Work out the finished part from the listing and answer in its coordinate system (mm). A direction names the side the tool comes from. Round coordinates to 2 decimals unless told otherwise and drop trailing zeros. Loops run counter-clockwise (first coordinate to the right, second up) from the corner with the lowest first, then second, coordinate; pieces in that order, holes last.
```python
from build123d import *

# Parameters (mm, degrees)
SKETCH_2_R          = 10
CUT_EXTRUDE_2_DEPTH = 13.84610836
CHAMFER_1_SIZE      = 0.3


with BuildPart() as part:
    # Эскиз1 → Повернуть1 (revolve)
    with BuildSketch(Plane(origin=(0, 0, 0), x_dir=(1, 0, 0), z_dir=(0, 1, 0)), mode=Mode.PRIVATE) as revolve_1_sk:
        Polygon((4.3, -7.45), (6.4, -7.45), (7.4, -6.45), (7.4, 0), (5.65, 0), (5.65, -5.75), (5.35, -5.75), (5.35, -6.8), (4.3, -6.8), align=None)
    revolve(revolve_1_sk.sketch.rotate(Axis((0, 0, 0), (0, 0, 1)), 180), axis=Axis((0, 0, 0), (0, 0, 1)))

    # Эскиз2 → Вырез-Вытянуть2 (cut, through all)
    with BuildSketch(Plane.XY):
        Circle(SKETCH_2_R)
        Polygon((8.082903769, 0), (4.041451884, 7), (-4.041451884, 7), (-8.082903769, 0), (-4.041451884, -7), (4.041451884, -7), align=None, mode=Mode.SUBTRACT)
    extrude(amount=CUT_EXTRUDE_2_DEPTH, mode=Mode.SUBTRACT)

    # Фаска1
    chamfer_1_edges = [part.edges().sort_by_distance(p)[0] for p in [
        (5.65, 0, 0),
    ]]
    chamfer(chamfer_1_edges, length=CHAMFER_1_SIZE)


solid = part.part
```
1. Determine the mould class of faces 3 (the face through (1.16, 5.223, 6.282)), 4 (the face through (-3.717, -6.399, 3.18)), 5 (the face through (3.717, 6.399, 3.18)) for opening direction Y: +Y half, -Y half, draft (parallel to the pull), parting line (faces both ways), or undercut.
Answer key:
face 3: undercut
face 4: -Y half
face 5: +Y half
2. Find section D-D (z = 6). Write down the section's boundary in (x, y).
Answer key:
outline: (-7.26, -1.42) - (-4.86, -5.58) arc R7.4 ccw to (-2.4, -7) - (2.4, -7) arc R7.4 ccw to (4.86, -5.58) - (7.26, -1.42) arc R7.4 ccw to (7.26, 1.42) - (4.86, 5.58) arc R7.4 ccw to (2.4, 7) - (-2.4, 7) arc R7.4 ccw to (-4.86, 5.58) - (-7.26, 1.42) arc R7.4 ccw to start; hole circle Ø10.7 at (0, 0)
3. Find section C-C (z = 2.75). Write down the section's boundary in (x, y), then the cut area to 3 significant figures.
Answer key:
outline: (-7.26, -1.42) - (-4.86, -5.58) arc R7.4 ccw to (-2.4, -7) - (2.4, -7) arc R7.4 ccw to (4.86, -5.58) - (7.26, -1.42) arc R7.4 ccw to (7.26, 1.42) - (4.86, 5.58) arc R7.4 ccw to (2.4, 7) - (-2.4, 7) arc R7.4 ccw to (-4.86, 5.58) - (-7.26, 1.42) arc R7.4 ccw to start; hole circle Ø11.3 at (0, 0)
area: 64.0 mm2
4. Given pin 1 (1.5 mm diameter, centred on y = 1.5, z = 6, fed in from +X); pin 2 (1.5 mm diameter, centred on x = 1.5, y = 1, fed in from -Z); pin 3 (1.5 mm diameter, centred on x = -5.5, y = -4, fed in from -Z); pin 4 (3 mm diameter, centred on y = 3.5, z = 6.5, fed in from +X), each flat-ended and moving along its own axis, determine where each tip first touches the part or whether it passes through.
Answer key:
pin 1: stops at x = 7.36
pin 2: passes through
pin 3: stops at z = 0
pin 4: stops at x = 6.93
5. Consider probe 1 along Y at (x, z) = (0, 6.5); probe 2 along Y at (x, z) = (-0.75, 3.75); probe 3 along Z at (x, y) = (-6.25, -3). Determine where each line is inside the solid, lowest interval first.
Answer key:
probe 1: y = -7 to -5.35, 5.35 to 7
probe 2: y = -7 to -5.6, 5.6 to 7
probe 3: z = 0 to 6.92
6. Which of the six approach directions +Z, -Z, +X, -X, +Y, -Y give full straight-line access (tool end or side, diameter ignored) to faces 1 (the face through (-5.39, -1.7, 3.06)), 2 (the face through (0, 7, 3))?
Answer key:
face 1: -Z
face 2: +Z, -Z, +X, -X, +Y
7. Find section B-B (y = 0). Write down the section's boundary in (x, z), then the cut area to 3 significant figures.
Answer key:
outline: (-7.4, 0) - (-5.95, 0) - (-5.65, 0.3) - (-5.65, 5.75) - (-5.35, 5.75) - (-5.35, 6.8) - (-4.3, 6.8) - (-4.3, 7.45) - (-6.4, 7.45) - (-7.4, 6.45) - close; (4.3, 6.8) - (5.35, 6.8) - (5.35, 5.75) - (5.65, 5.75) - (5.65, 0.3) - (5.95, 0) - (7.4, 0) - (7.4, 6.45) - (6.4, 7.45) - (4.3, 7.45) - close
area: 27.4 mm2
8. Find section A-A (x = 0). Write down the section's boundary in (y, z), then the cut area to 4 significant figures.
Answer key:
outline: (-7, 0) - (-5.95, 0) - (-5.65, 0.3) - (-5.65, 5.75) - (-5.35, 5.75) - (-5.35, 6.8) - (-4.3, 6.8) - (-4.3, 7.45) - (-6.4, 7.45) - (-7, 6.85) - close; (4.3, 6.8) - (5.35, 6.8) - (5.35, 5.75) - (5.65, 5.75) - (5.65, 0.3) - (5.95, 0) - (7, 0) - (7, 6.85) - (6.4, 7.45) - (4.3, 7.45) - close
area: 22.05 mm2
